For this review, use the dimensioned drawing (mm, ordinates from the lowest corner) and the shaded views. A direction names the side the tool comes from. Give positions to 0.01 mm unless a question says otherwise; leave off trailing zeros. Loops run counter-clockwise (first coordinate to the right, second up) from the corner with the lowest first, then second, coordinate; pieces in that order, holes last. Notation, with made-up numbers: M 86.25,-17.5 L 107.25,-17.5 A19 cw 107.25,-0.5 Z; hole C 83,-3.5 d8. An arc over 180 degrees is marked long. Use CSV: the item, a comma, the result in double quotes. Start each with the question number.
1. Take a section at C-C, the plane z = 17.5. Write out the cut boundary in (x, y).
2. Tool access review of the marked faces 4 and 5: name each direction out of +Z, -Z, +X, -X, +Y, -Y from which nothing blocks a thin tool from reaching the whole face with its end or side.
3. Take a section at D-D, the plane y = 20. Write out the cut boundary in (x, z).
4. The part is to be moulded in two halves that separate along Y. For the marked faces 1, 2 and 3, say which applies: pulls with the +Y half, pulls with the -Y half, needs draft (parallel to the pull), parting line crosses it, or undercut.
5. Take a section at A-A, the plane y = 5. Write out the cut boundary in (x, z), and give its area (4 significant figures).
6. Take a section at B-B, the plane x = 11.25. Write out the cut boundary in (y, z).
7. To check wall thickness, follow line 1 (Y direction, x = 13.55, z = 10); line 2 (Y direction, x = 2.25, z = 17.5); line 3 (Z direction, x = 14, y = 10). State the ranges of each line that lie inside material, in increasing order. Write a range as [from, to].
8. Insertion check: P1, Ø2.5, axis at x = 3, y = 30, coming from the -Z side; P2, Ø3.5, axis at y = 16, z = 8, coming from the -X side; P3, Ø2.5, axis at y = 27.5, z = 16.5, coming from the -X side; P4, Ø5, axis at x = 3, y = 12, coming from the -Z side. Each pin has a flat end and moves straight along its axis. Give the tip position at first contact, or say it passes through.
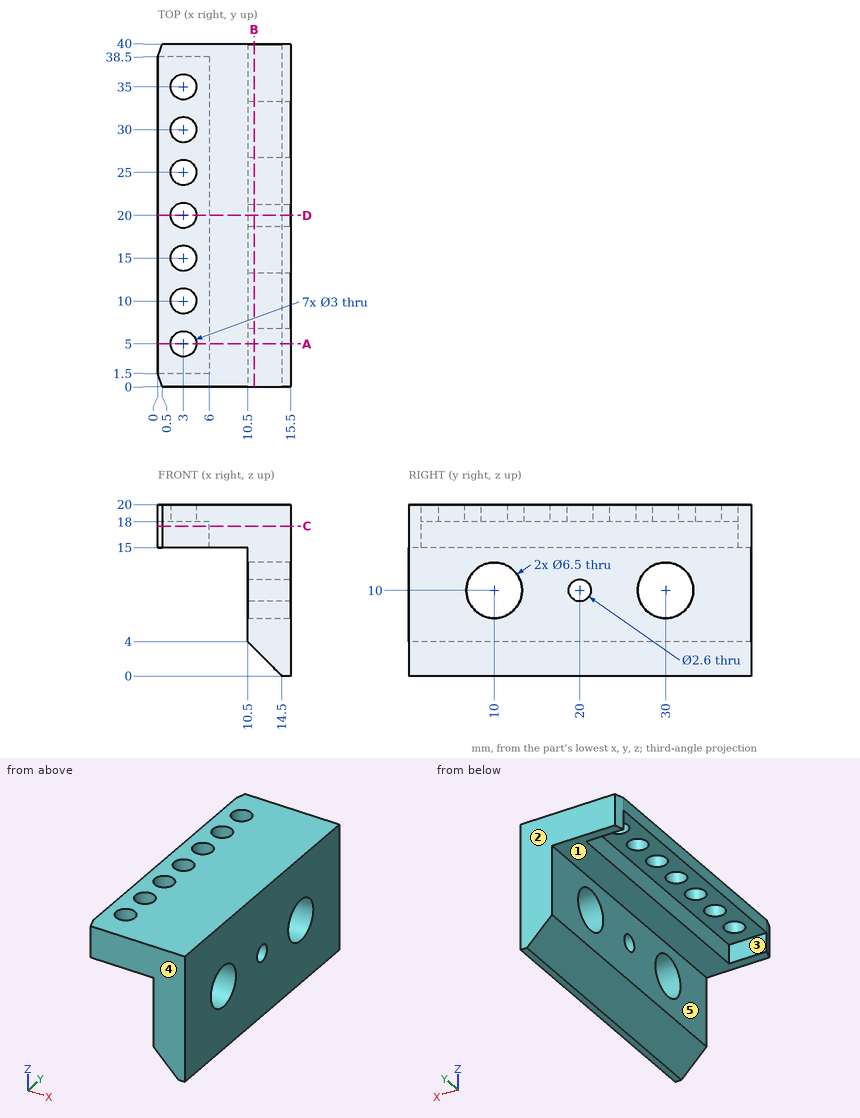
Result set:
1,outline,"M 0,1.5 L 0.5,0 L 15.5,0 L 15.5,40 L 0.5,40 L 0,38.5 L 6,38.5 L 6,1.5 Z"
2,face 4,"+Z, -Z, +X, -X, -Y"
2,face 5,"-Z, -X, +Y, -Y"
3,outline,"M 0,18 L 1.5,18 L 1.5,20 L 0,20 Z; M 4.5,18 L 6,18 L 6,15 L 10.5,15 L 10.5,11.3 L 15.5,11.3 L 15.5,20 L 4.5,20 Z; M 10.5,4 L 14.5,0 L 15.5,0 L 15.5,8.7 L 10.5,8.7 Z"
4,face 1,"needs draft"
4,face 2,"pulls with the +Y half"
4,face 3,"undercut"
5,outline,"M 0,18 L 1.5,18 L 1.5,20 L 0,20 Z; M 4.5,18 L 6,18 L 6,15 L 10.5,15 L 10.5,4 L 14.5,0 L 15.5,0 L 15.5,20 L 4.5,20 Z"
5,area,"120.5 mm2"
6,outline,"M 0,3.25 L 40,3.25 L 40,20 L 0,20 Z; hole C 10,10 d6.5; hole C 20,10 d2.6; hole C 30,10 d6.5"
7,line 1,"[0, 6.75], [13.25, 18.7], [21.3, 26.75], [33.25, 40]"
7,line 2,"[0, 1.5], [38.5, 40]"
7,line 3,"[0.5, 6.75], [13.25, 20]"
8,P1,"through"
8,P2,"x = 10.5"
8,P3,"x = 6"
8,P4,"z = 18"
